Part model, mm, in its own coordinate system. Round coordinates to 2 decimals unless told otherwise and drop trailing zeros. Order: outer loops, then holes, each group sorted by start corner. A loop starts at its lowest first (then second) coordinate and runs counter-clockwise, first axis right, second up. Notation, with made-up numbers: (-23.5, 35.25) -> (35.5, 35.25) arc R28 cw to (35.5, 67.25) -> close; hole circle Ø1 at (12.25, -15). An arc over 180 degrees is marked (long way). Use CSV: the item, a comma, the result in double quotes.
```python
from build123d import *

# Parameters (mm, degrees)
SKETCH1_W           = 81.8
SKETCH1_H           = 102
BOSS_EXTRUDE1_DEPTH = 1.5
SKETCH2_W           = 10.6
SKETCH2_H           = 3
SKETCH2_W_2         = 6.445
SKETCH2_R           = 1.5
CUT_EXTRUDE1_DEPTH  = 2.5
FILLET1_R           = 5


with BuildPart() as part:
    # Sketch1 → Boss-Extrude1 (new body)
    with BuildSketch(Plane.XY):
        with Locations((40.9, 51)):
            Rectangle(SKETCH1_W, SKETCH1_H)
    extrude(amount=BOSS_EXTRUDE1_DEPTH)

    # Sketch2 → Cut-Extrude1 (cut, through all)
    with BuildSketch(Plane.XY.offset(1.5)):
        with Locations((5.3, 1.5)):
            Rectangle(SKETCH2_W, SKETCH2_H)
        with Locations((44.1225, 1.5)):
            Rectangle(SKETCH2_W_2, SKETCH2_H)
        with Locations((37.6775, 1.5)):
            Rectangle(SKETCH2_W_2, SKETCH2_H)
        with Locations((76.5, 1.5)):
            Rectangle(SKETCH2_W, SKETCH2_H)
        with Locations((6, 96)):
            Circle(SKETCH2_R)
        with Locations((75.8, 96)):
            Circle(SKETCH2_R)
    extrude(amount=-CUT_EXTRUDE1_DEPTH, mode=Mode.SUBTRACT)

    # Fillet1
    fillet1_edges = [part.edges().sort_by_distance(p)[0] for p in [
        (0, 102, 0.75),
        (81.8, 102, 0.75),
    ]]
    fillet(fillet1_edges, radius=FILLET1_R)


solid = part.part
```
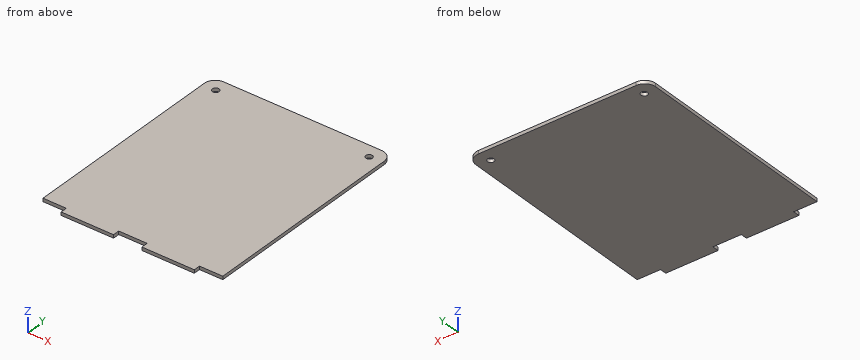
(1) Probe probe 1 along X at (y, z) = (96, 0.5); probe 2 along Y at (x, z) = (6, 0.8); probe 3 along Y at (x, z) = (4, 0.65). List the from-to ranges inside material, lowest first. Write a range as [from, to].
Reply:
probe 1,"[0, 4.5], [7.5, 74.3], [77.3, 81.8]"
probe 2,"[3, 94.5], [97.5, 102]"
probe 3,"[3, 101.9]"
(2) Drop flat-ended pins along their axis: P1, Ø0.8, axis at y = 1.5, z = 1, coming from the -X side; P2, Ø1.8, axis at x = 75.8, y = 96, coming from the +Z side; P3, Ø0.8, axis at y = 1, z = 1, coming from the +X side. Give the stop position or say it passes through.
Reply:
P1,"x = 10.6"
P2,"through"
P3,"x = 71.2"
(3) Cut at A-A, the plane z = 0.75. Give the cut face in (x, y) (3 decimals).
Reply:
outline,"(0, 3) -> (10.6, 3) -> (10.6, 0) -> (34.455, 0) -> (34.455, 3) -> (47.345, 3) -> (47.345, 0) -> (71.2, 0) -> (71.2, 3) -> (81.8, 3) -> (81.8, 97) arc R5 ccw to (76.8, 102) -> (5, 102) arc R5 ccw to (0, 97) -> close; hole circle Ø3 at (6, 96); hole circle Ø3 at (75.8, 96)"
(4) Cut at B-B, the plane x = 40.5. Give the cut face in (y, z).
Reply:
outline,"(3, 0) -> (102, 0) -> (102, 1.5) -> (3, 1.5) -> close"
